from build123d import *

# Parameters (mm, degrees)
SKETCH1_W                               = 20
SKETCH1_H                               = 20
BOSS_EXTRUDE1_DEPTH                     = 10
SKETCH2_R                               = 8
CUT_EXTRUDE2_DEPTH                      = 46
SKETCH3_R                               = 4
SKETCH3_R_2                             = 4.5
CUT_EXTRUDE3_DEPTH                      = 10
CBORE_FOR_M5_HEX_HEAD_BOLT1_D           = 4
CBORE_FOR_M5_HEX_HEAD_BOLT1_DEPTH       = 10
CBORE_FOR_M5_HEX_HEAD_BOLT1_CBORE_D     = 7
CBORE_FOR_M5_HEX_HEAD_BOLT1_CBORE_DEPTH = 1
CBORE_FOR_M5_HEX_HEAD_BOLT2_D           = 4
CBORE_FOR_M5_HEX_HEAD_BOLT2_DEPTH       = 10
CBORE_FOR_M5_HEX_HEAD_BOLT2_CBORE_D     = 7
CBORE_FOR_M5_HEX_HEAD_BOLT2_CBORE_DEPTH = 1
CUT_EXTRUDE4_DEPTH                      = 2
CUT_EXTRUDE5_DEPTH                      = 1
CUT_EXTRUDE6_DEPTH                      = 2
CUT_EXTRUDE7_DEPTH                      = 1


with BuildPart() as part:
    # Sketch1 → Boss-Extrude1 (new body)
    with BuildSketch(Plane(origin=(0, 0, 0), x_dir=(1, 0, 0), z_dir=(0, 1, 0))):
        with BuildLine():
            Line((23.939871077, 2.849965846), (42.576368333, -0.125028462))
            ThreePointArc((42.576368333, -0.125028462), (51, -10), (42.576368333, -19.874971538))
            Line((42.576368333, -19.874971538), (30.130588759, -21.86172489))
            ThreePointArc((30.130588759, -21.86172489), (24.291669579, -24.533541475), (20.666245259, -29.833341429))
            Line((20.666245259, -29.833341429), (15.677992749, -44.439174654))
            ThreePointArc((15.677992749, -44.439174654), (10, -48.5), (4.322007251, -44.439174654))
            Line((4.322007251, -44.439174654), (-2.355985499, -24.885704137))
            ThreePointArc((-2.355985499, -24.885704137), (-2.837901545, -22.973082941), (-3, -21.00735483))
            Line((-3, -21.00735483), (-3, 1))
            ThreePointArc((-3, 1), (-2.414213562, 2.414213562), (-1, 3))
            Line((-1, 3), (22.048229077, 3))
            ThreePointArc((22.048229077, 3), (22.997020375, 2.962432657), (23.939871077, 2.849965846))
        make_face()
        with Locations((10, -10)):
            Rectangle(SKETCH1_W, SKETCH1_H, mode=Mode.SUBTRACT)
    extrude(amount=BOSS_EXTRUDE1_DEPTH)

    # Sketch2 → Cut-Extrude2 (cut)
    with BuildSketch(Plane(origin=(0, 5, 0), x_dir=(1, 0, 0), z_dir=(0, 1, 0))):
        with Locations(Location((41, -10, 0), (0, 0, 90))):
            Circle(SKETCH2_R)
    extrude(amount=CUT_EXTRUDE2_DEPTH, mode=Mode.SUBTRACT)

    # Sketch3 → Cut-Extrude3 (cut)
    with BuildSketch(Plane(origin=(0, 5, 0), x_dir=(1, 0, 0), z_dir=(0, 1, 0))):
        with Locations(Location((10, -42.5, 0), (0, 0, 90))):
            Circle(SKETCH3_R)
        with Locations(Location((41, -10, 0), (0, 0, 90))):
            Circle(SKETCH3_R_2)
    extrude(amount=-CUT_EXTRUDE3_DEPTH, mode=Mode.SUBTRACT)

    # CBORE for M5 Hex Head Bolt1
    with Locations(Plane.ZY.offset(3)):
        with Locations((10, 5)):
            CounterBoreHole(CBORE_FOR_M5_HEX_HEAD_BOLT1_D / 2, CBORE_FOR_M5_HEX_HEAD_BOLT1_CBORE_D / 2, CBORE_FOR_M5_HEX_HEAD_BOLT1_CBORE_DEPTH, depth=CBORE_FOR_M5_HEX_HEAD_BOLT1_DEPTH)

    # CBORE for M5 Hex Head Bolt2
    with Locations(Plane(origin=(0, 0, -3), x_dir=(-1, 0, 0), z_dir=(0, 0, -1))):
        with Locations((-10, 5)):
            CounterBoreHole(CBORE_FOR_M5_HEX_HEAD_BOLT2_D / 2, CBORE_FOR_M5_HEX_HEAD_BOLT2_CBORE_D / 2, CBORE_FOR_M5_HEX_HEAD_BOLT2_CBORE_DEPTH, depth=CBORE_FOR_M5_HEX_HEAD_BOLT2_DEPTH)

    # Sketch9 → Cut-Extrude4 (cut)
    with BuildSketch(Plane(origin=(0, 0, -2), x_dir=(-1, 0, 0), z_dir=(0, 0, -1))):
        Polygon((-10, 2.5), (-8.8, 3.4), (-11.2, 3.4), align=None)
    extrude(amount=-CUT_EXTRUDE4_DEPTH, mode=Mode.SUBTRACT)

    # Sketch10 → Cut-Extrude5 (cut)
    with BuildSketch(Plane(origin=(0, 0, -2), x_dir=(-1, 0, 0), z_dir=(0, 0, -1))):
        Polygon((-10, 0.5), (-7.800112236, 2.277777778), (-12.199887764, 2.277777778), align=None)
    extrude(amount=CUT_EXTRUDE5_DEPTH, mode=Mode.SUBTRACT)

    # Sketch11 → Cut-Extrude6 (cut)
    with BuildSketch(Plane.ZY.offset(2)):
        Polygon((10, 2.5), (11.2, 3.4), (8.8, 3.4), align=None)
    extrude(amount=-CUT_EXTRUDE6_DEPTH, mode=Mode.SUBTRACT)

    # Sketch13 → Cut-Extrude7 (cut)
    with BuildSketch(Plane.ZY.offset(2)):
        Polygon((10, 0.5), (7.800112236, 2.277777778), (12.199887764, 2.277777778), align=None)
    extrude(amount=CUT_EXTRUDE7_DEPTH, mode=Mode.SUBTRACT)


solid = part.part
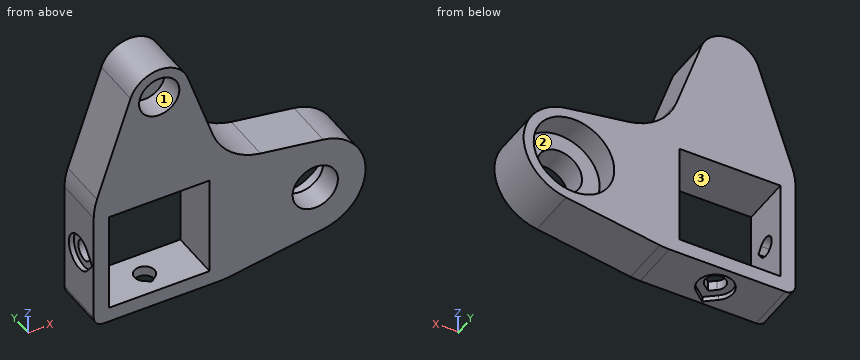
Check sheet for the modelled part. Datum: model origin and axes. Units: mm. Face numbers are marked on the shaded views. A direction names the side the tool comes from. Give positions to 0.01 mm unless a question says otherwise; leave off trailing zeros. Write each loop counter-clockwise with the first axis right and the second up, starting at its lowest first coordinate (ties: lowest second). Pieces come first, ordered by that corner, then holes. Notation, with made-up numbers: (-36, 12) -> (2, 12) arc R29 ccw to (2, 47) -> close; hole circle Ø10 at (42.25, 3.25). An arc over 180 degrees is marked (long way). One line per item, written item: value. Start each with the question number.
Item 1: Section check A-A on x = 17. Record the cut outline in (y, z).
Item 2: Section check C-C on x = 46.5. Record the cut outline in (y, z), then the cut area to 3 significant figures.
Item 3: Section check D-D on z = 42.5. Record the cut outline in (x, y), then the cut area to 3 significant figures.
Item 4: Material ranges on probe 1 along X at (y, z) = (7.15, 10); probe 2 along X at (y, z) = (8.85, 10); probe 3 along Y at (x, z) = (-2.5, 10), recorded low to high. Write a range as from..to.
Item 5: Tool access check on the marked faces 1, 2 and 3. Record the directions out of +Z, -Z, +X, -X, +Y, -Y that give a thin tool (end or side, any length) a straight path to the whole face; none if there is none.
Item 6: Section check B-B on z = 4.5. Record the cut outline in (x, y), then the cut area to 3 significant figures.
Item 7: Gauge pin test, flat ends, axial feed: pin 1 (2 mm diameter, centred on y = 5.5, z = 10.5, fed in from -X); pin 2 (8 mm diameter, centred on x = 38.5, z = 11, fed in from +Y); pin 3 (1 mm diameter, centred on y = 8, z = 38, fed in from -X). Record the tip position at first contact, or that the pin passes through.
Results list:
1. outline: (0, -3) -> (10, -3) -> (10, 0) -> (0, 0) -> close; (0, 20) -> (10, 20) -> (10, 40.57) -> (0, 40.57) -> close
2. outline: (0, 1.65) -> (10, 1.65) -> (10, 4.19) -> (5, 4.19) -> (5, 15.81) -> (10, 15.81) -> (10, 18.35) -> (0, 18.35) -> close
2. area: 109 mm²
3. outline: (3.66, 0) -> (6, 0) -> (6, 5) -> (14, 5) -> (14, 0) -> (16.34, 0) -> (16.34, 10) -> (3.66, 10) -> close
3. area: 86.8 mm²
4. probe 1: -2..0, 20..33, 49..51
4. probe 2: -3..0, 20..33, 49..51
4. probe 3: 0..0.5, 8.5..10
5. face 1: -Y
5. face 2: +Y
5. face 3: +Y, -Y
6. outline: (-3, 0) -> (0, 0) -> (0, 10) -> (-3, 10) -> close; (20, 0) -> (49.35, 0) -> (49.35, 10) -> (46.81, 10) -> (46.81, 5) -> (35.19, 5) -> (35.19, 10) -> (20, 10) -> close
6. area: 265 mm²
7. pin 1: x = 20
7. pin 2: y = 5
7. pin 3: x = 1.95
